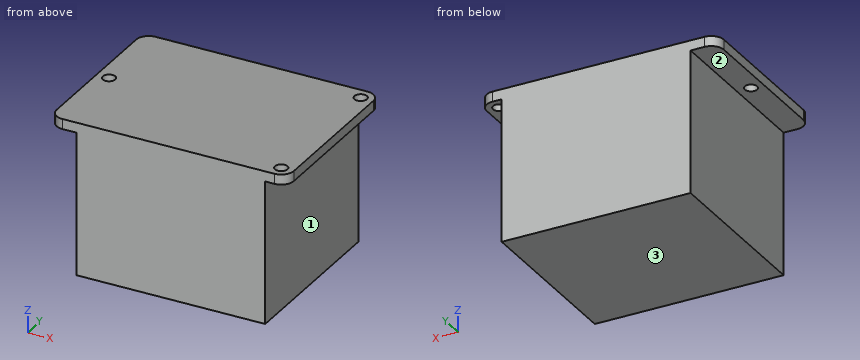
```python
from build123d import *

# Parameters (mm, degrees)
SKETCH_1_W               = 56.5
SKETCH_1_H               = 41
EXTRUDE_1_DEPTH          = 2.4
CUT_EXTRUDE_1_DEPTH      = 70.849910522
CUT_EXTRUDE_1_DEPTH_BACK = 70.849910522
SKETCH_2_R               = 1.5
SKETCH_3_W               = 45
SKETCH_3_H               = 41
EXTRUDE_2_DEPTH          = 34
FILLET_1_R               = 3


with BuildPart() as part:
    # 草图1 → 凸台-拉伸1 (new body)
    with BuildSketch(Plane.XY):
        with Locations((28.25, -20.5)):
            Rectangle(SKETCH_1_W, SKETCH_1_H)
    extrude(amount=EXTRUDE_1_DEPTH)

    # 草图2 → 切除-拉伸1 (cut, two sides: drawn at the far end of the back side and taken through both)
    with BuildSketch(Plane.XY.offset(2.4).offset(-CUT_EXTRUDE_1_DEPTH_BACK)):
        with Locations((53.5, -3)):
            Circle(SKETCH_2_R)
        with Locations((53.5, -38)):
            Circle(SKETCH_2_R)
        with Locations((3, -20.5)):
            Circle(SKETCH_2_R)
    extrude(amount=CUT_EXTRUDE_1_DEPTH + CUT_EXTRUDE_1_DEPTH_BACK, mode=Mode.SUBTRACT)

    # 草图3 → 凸台-拉伸2 (add)
    with BuildSketch(Plane(origin=(0, 0, 0), x_dir=(-1, 0, 0), z_dir=(0, 0, -1))):
        with Locations((-28.809280121, -20.5)):
            Rectangle(SKETCH_3_W, SKETCH_3_H)
    extrude(amount=EXTRUDE_2_DEPTH)

    # 圆角1
    fillet_1_edges = [part.edges().sort_by_distance(p)[0] for p in [
        (0, 0, 1.2),
        (56.5, 0, 1.2),
        (56.5, -41, 1.2),
        (0, -41, 1.2),
    ]]
    fillet(fillet_1_edges, radius=FILLET_1_R)


solid = part.part
```
Model file for the job. Use its own axes, mm. Face numbers are marked on the shaded views. A direction names the side the tool comes from. Coordinates: 2 decimals unless noted, no trailing zeros. Loops run counter-clockwise (first coordinate to the right, second up) from the corner with the lowest first, then second, coordinate; pieces in that order, holes last. Notation, with made-up numbers: (80.25, -17) - (87.25, -17) arc R30 ccw to (87.25, 5) - close; hole circle Ø10 at (24, -1.75). An arc over 180 degrees is marked (long way). Answer as a JSON object with one key per item and string values. Group by question number.
(1) Probe line 1 along Y through (x, z) = (53, 1); line 2 along X through (y, z) = (-38, 1.3); line 3 along Y through (x, z) = (3, 1.5). List the from-to ranges inside material, lowest first.
(2) Tool access for the marked faces 1, 2 and 3: list every direction of +Z, -Z, +X, -X, +Y, -Y with a clear straight run to the whole face (end or side of a thin tool).
(3) Flat gauge pins, fed straight in: pin 1 (3 mm diameter, centred on x = 31, z = -30.5, fed in from +Y); pin 2 (2.5 mm diameter, centred on x = 53.5, y = -3, fed in from -Z); pin 3 (3 mm diameter, centred on x = 4, y = -21.5, fed in from -Z); pin 4 (4 mm diameter, centred on y = -6, z = -7, fed in from -X). Where does each tip first touch, or does it go through?
(4) Cut at B-B (z = -23). Give the cut face in (x, y), then the cut area to 4 significant figures.
(5) Cut at A-A (y = -25.5). Give the cut face in (x, z), then the cut area to 3 significant figures.
Geometry says:
{
 "1": {"line 1": "y = -41 to -39.41, -36.59 to -4.41, -1.59 to 0", "line 2": "x = 0 to 52, 55 to 56.5", "line 3": "y = -41 to -22, -19 to 0"},
 "2": {"face 1": "-Z, +X, +Y, -Y", "face 2": "-Z, -X, +Y, -Y", "face 3": "-Z, +X, -X, +Y, -Y"},
 "3": {"pin 1": "stops at y = 0", "pin 2": "passes through", "pin 3": "stops at z = 0", "pin 4": "stops at x = 6.31"},
 "4": {"outline": "(6.31, -41) - (51.31, -41) - (51.31, 0) - (6.31, 0) - close", "area": "1,845 mm^2"},
 "5": {"outline": "(0, 0) - (6.31, 0) - (6.31, -34) - (51.31, -34) - (51.31, 0) - (56.5, 0) - (56.5, 2.4) - (0, 2.4) - close", "area": "1,670 mm^2"}
}
